Geometry: final body of the model. Coordinates: model frame, mm. Face numbers are marked on the shaded views. Give positions to 0.01 mm unless a question says otherwise; leave off trailing zeros. Write each loop counter-clockwise with the first axis right and the second up, starting at its lowest first coordinate (ties: lowest second). Pieces come first, ordered by that corner, then holes.
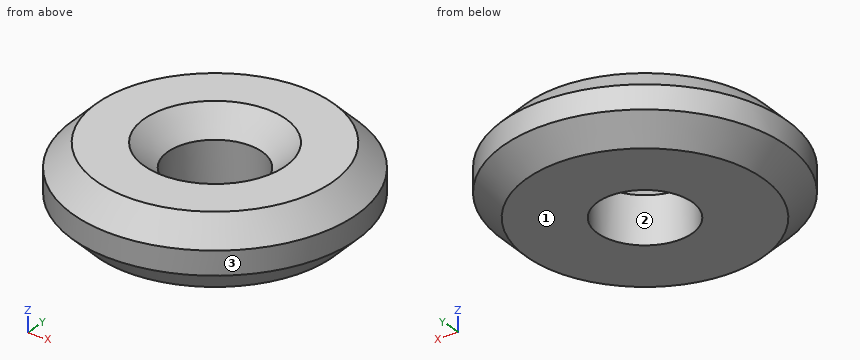
```python
from build123d import *

# Parameters (mm, degrees)
ESQUISSE1_R             = 6
BASE_EXTRUSION_DEPTH    = 3
CHANFREIN1_SIZE         = 1
ESQUISSE2_R             = 2
ENL_V_MAT_EXTRU_1_DEPTH = 10
CHANFREIN3_SIZE         = 1


with BuildPart() as part:
    # Esquisse1 → Base-Extrusion (new body)
    with BuildSketch(Plane.XY):
        Circle(ESQUISSE1_R)
    extrude(amount=-BASE_EXTRUSION_DEPTH)

    # Chanfrein1
    chanfrein1_edges = [part.edges().sort_by_distance(p)[0] for p in [
        (-6, 0, 0),
        (-6, 0, -3),
    ]]
    chamfer(chanfrein1_edges, length=CHANFREIN1_SIZE)

    # Esquisse2 → Enlèv. mat.-Extru.1 (cut, through all)
    with BuildSketch(Plane.XY):
        Circle(ESQUISSE2_R)
    extrude(amount=-ENL_V_MAT_EXTRU_1_DEPTH, mode=Mode.SUBTRACT)

    # Chanfrein3
    chanfrein3_edges = [part.edges().sort_by_distance(p)[0] for p in [
        (-2, 0, 0),
    ]]
    chamfer(chanfrein3_edges, length=CHANFREIN3_SIZE)


solid = part.part
```
Item 1: Section C-C, the plane z = -2.6. Return the cut outline in (x, y).
Found:
outline: circle Ø10.8 at (0, 0); hole circle Ø4 at (0, 0)
Item 2: Line query: L1, parallel to Y at x = 0, z = -1.7; L2, parallel to Y at x = -1, z = -0.65; L3, parallel to X at y = -2.25, z = -0.5. Output: solid intervals per line, ascending.
Found:
L1: y = -6 to -2, 2 to 6
L2: y = -5.56 to -2.13, 2.13 to 5.56
L3: x = -5.02 to -1.09, 1.09 to 5.02
Item 3: Pin query (flat end, axial travel): pin 1 Ø2.5 at (x, y) = (0, 0) entering from -Z; pin 2 Ø1 at (y, z) = (2, -1.5) entering from +X. Return the tip coordinate at first contact, or that it passes through.
Found:
pin 1: passes through
pin 2: stops at x = 5.81
Item 4: Pull-direction query (X, two-part tool) for the marked faces 1, 2 and 3; classes: +X half, -X half, draft (parallel to the pull), parting line (faces both ways), or undercut.
Found:
face 1: draft
face 2: undercut
face 3: parting line
Item 5: Section D-D, the plane z = -0.45. Return the cut outline in (x, y).
Found:
outline: circle Ø10.9 at (0, 0); hole circle Ø5.1 at (0, 0)
Item 6: Section A-A, the plane x = 0. Return the cut outline in (y, z).
Found:
outline: (-6, -2) - (-5, -3) - (-2, -3) - (-2, -1) - (-3, 0) - (-5, 0) - (-6, -1) - close; (2, -3) - (5, -3) - (6, -2) - (6, -1) - (5, 0) - (3, 0) - (2, -1) - close
